Input: part model. Units: mm. Frame: model coordinates. A direction names the side the tool comes from. Round coordinates to 2 decimals unless told otherwise and drop trailing zeros. Answer as a JSON object with one key per item and string values.
```python
from build123d import *

# Parameters (mm, degrees)
M16_TAPPED_HOLE1_D     = 14
M16_TAPPED_HOLE1_DEPTH = 35
M16_TAPPED_HOLE1_TIP   = 4.206024333
CUT_EXTRUDE1_DEPTH     = 1
CIRPATTERN1_COUNT      = 8
FILLET1_R              = 3


with BuildPart() as part:
    # Sketch3 → Revolve1 (revolve)
    with BuildSketch(Plane.XY, mode=Mode.PRIVATE) as revolve1_sk:
        with BuildLine():
            Line((0, 0), (22, 0))
            Line((22, 0), (22, 4))
            Line((22, 4), (19, 4))
            Line((19, 4), (19, 10))
            Line((19, 10), (30, 10))
            Line((30, 10), (30, 40))
            ThreePointArc((30, 40), (15.811388301, 47.434164903), (0, 50))
            Line((0, 50), (0, 0))
        make_face()
    revolve(revolve1_sk.sketch.rotate(Axis((0, 0, 0), (0, 1, 0)), 90), axis=Axis((0, 0, 0), (0, 1, 0)))

    # M16 Tapped Hole1
    with Locations(Plane.XZ):
        with Locations((0, 0)):
            Hole(M16_TAPPED_HOLE1_D / 2, depth=M16_TAPPED_HOLE1_DEPTH)
            with Locations((0, 0, -(M16_TAPPED_HOLE1_DEPTH + M16_TAPPED_HOLE1_TIP / 2))):  # 118° drill point
                Cone(0, M16_TAPPED_HOLE1_D / 2, M16_TAPPED_HOLE1_TIP, mode=Mode.SUBTRACT)

    # Sketch7 → Cut-Extrude1 (cut, symmetric)
    with BuildSketch(Plane.XY):
        Polygon((30, 40), (30, 10), (19, 10), align=None)
    cut_extrude1 = extrude(amount=CUT_EXTRUDE1_DEPTH, both=True, mode=Mode.SUBTRACT)

    # CirPattern1: Cut-Extrude1 ×8 about axis
    cirpattern1_axis = Axis((0, 0, 0), (0, 1, 0))
    for i in range(1, CIRPATTERN1_COUNT):
        add(cut_extrude1.rotate(cirpattern1_axis, i * 360 / CIRPATTERN1_COUNT), mode=Mode.SUBTRACT)

    # Fillet1
    fillet1_edges = [part.edges().sort_by_distance(p)[0] for p in [
        (27.716385975, 10, 11.480502971),
        (11.480502971, 10, 27.716385975),
        (-11.480502971, 10, 27.716385975),
        (-27.716385975, 10, 11.480502971),
        (-27.716385975, 10, -11.480502971),
        (-11.480502971, 10, -27.716385975),
        (11.480502971, 10, -27.716385975),
        (27.716385975, 10, -11.480502971),
    ]]
    fillet(fillet1_edges, radius=FILLET1_R)


solid = part.part
```
1) Reachability of faces 1 (the face through (17.26, 24.79, 17.28)), 2 (the face through (-11.633, 26.689, 27.653)), 3 (the face through (9, 10, -20)), 4 (the face through (-6.466, 17.745, -2.681)), 5 (the face through (-9, 10, -22)) from +Z, -Z, +X, -X, +Y, -Y: full face, straight path, thin tool, end or side. Return the list, or none.
Output:
{"face 1": "none", "face 2": "+Z, -X, +Y, -Y", "face 3": "-Z, +X", "face 4": "-Y", "face 5": "-Z, -X"}
2) Contact query for flat-ended pins moving along their axis: P1, Ø1.5, axis at x = 17.5, y = 14.5, coming from the -Z side; P2, Ø9, axis at y = 27, z = -22.5, coming from the -X side; P3, Ø5.5, axis at y = 28, z = 26.5, coming from the +X side. Output: stop coordinate, or through.
Output:
{"P1": "stops at z = -24.89", "P2": "stops at x = -24", "P3": "stops at x = 18.33"}
3) Draft query along X for faces 6 (the face through (24.423, 24.79, 0.014)), 7 (the face through (-19.806, 18.53, -18.391)), 8 (the face through (27, 19, 1)). Return one class per face: +X half, -X half, draft (parallel to the pull), parting line (faces both ways), or undercut.
Output:
{"face 6": "+X half", "face 7": "undercut", "face 8": "draft"}
4) Ray query, probe 1 along X at (y, z) = (9, 0); probe 2 along Z at (x, y) = (18, 26); probe 3 along Z at (x, y) = (0, 22). Return the intervals inside material, ascending.
Output:
{"probe 1": "x = -19 to -7, 7 to 19", "probe 2": "z = -24 to -19.41, -17.17 to 17.17, 19.41 to 24", "probe 3": "z = -23.4 to -7, 7 to 23.4"}
